The listing builds one solid part. Answer for the finished solid, in the listing's coordinates (mm). Face numbers are marked on the shaded views. A direction names the side the tool comes from. Coordinates: 2 decimals unless noted, no trailing zeros. Write each loop counter-clockwise with the first axis right and the second up, starting at its lowest first coordinate (ties: lowest second). Pieces come first, ordered by that corner, then holes.
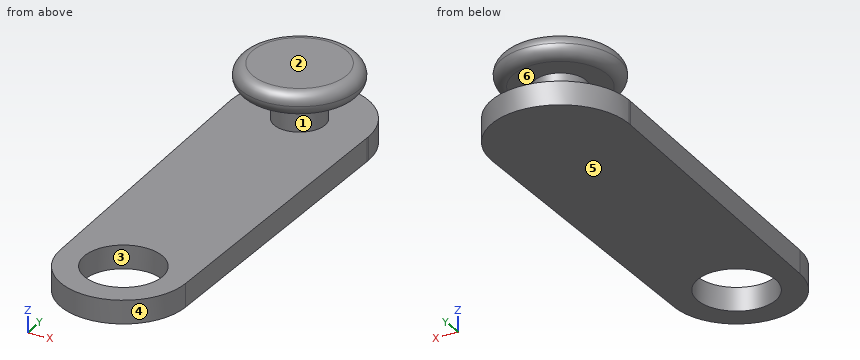
from build123d import *

# Parameters (mm, degrees)
F0_R     = 5
F1_DEPTH = 3
F2_R     = 3.25
F3_DEPTH = 4
F4_R     = 7.5
F5_DEPTH = 3
F6_R     = 1.49999


# Not quite as in the source:
# - a fillet or chamfer is up to 0.001 mm smaller than in the source, because OpenCascade refuses the exact size


with BuildPart() as f1:
    # F0 (on Top) → F1 (new body)
    with BuildSketch(Plane.XY):
        with BuildLine():
            Line((8.8034559258, 0), (8.7968361379, -0.3413359058))
            ThreePointArc((8.7968361379, -0.3413359058), (8.8018008233, -0.1707000455), (8.8034559258, 0))
        make_face()
        with BuildLine():
            Line((8.024687147, -40.1556288865), (8.7968361379, -0.3413359058))
            Line((8.7968361379, -0.3413359058), (8.8034559258, 0))
            ThreePointArc((8.8034559258, 0), (0, 8.8034559258), (-8.8034559258, 0))
            Line((-8.8034559258, 0), (-8.7968361379, -0.3413359058))
            Line((-8.7968361379, -0.3413359058), (-8.024687147, -40.1556288865))
            ThreePointArc((-8.024687147, -40.1556288865), (0, -48.02619612), (8.024687147, -40.1556288865))
        make_face()
        with Locations((0, -40)):
            Circle(F0_R, mode=Mode.SUBTRACT)
        with BuildLine():
            Line((-8.7968361379, -0.3413359058), (-8.8034559258, 0))
            ThreePointArc((-8.8034559258, 0), (-8.8018008233, -0.1707000455), (-8.7968361379, -0.3413359058))
        make_face()
    extrude(amount=F1_DEPTH)

    # F2 (on face) → F3 (join)
    with BuildSketch(Plane.XY.offset(3)):
        Circle(F2_R)
    extrude(amount=F3_DEPTH)

    # F4 (on face) → F5 (join)
    with BuildSketch(Plane.XY.offset(7)):
        Circle(F4_R)
    extrude(amount=F5_DEPTH)

    # F6 (radius 1.5 in the source; OpenCascade refuses exactly that, so slightly less here)
    f6_edges = [f1.edges().sort_by_distance(p)[0] for p in [
        (-7.5, 0, 10),
        (-7.5, 0, 7),
    ]]
    fillet(f6_edges, radius=F6_R)


solid = f1.part
1. For a pull along Y with two mould halves and no side action, classify the marked faces 1, 2, 3 and 4 as pulls with the +Y half, pulls with the -Y half, needs draft (parallel to the pull), parting line crosses it, or undercut.
Results found:
face 1: parting line crosses it
face 2: needs draft
face 3: undercut
face 4: pulls with the -Y half
2. A tool of negligible diameter and unlimited length cuts with its end or side. For the marked faces 5 and 6, from which of +Z, -Z, +X, -X, +Y, -Y can it reach the whole face along a straight path? Write none if from no direction.
Results found:
face 5: -Z, +X, -X, +Y, -Y
face 6: none
3. Section C-C on y = -34.5 is taken. Give the vertices of the cut face in (x, z).
Results found:
outline: (-8.13, 0) - (8.13, 0) - (8.13, 3) - (-8.13, 3) - close
4. Flat-ended cylindrical pins translate along their axes: P1, Ø4, axis at x = 1.5, z = 7, coming from the -Y side; P2, Ø9, axis at x = 0, y = -20.5, coming from the +Z side; P3, Ø1, axis at x = -5, z = 2.5, coming from the +Y side; P4, Ø3, axis at x = 7, y = -18, coming from the -Z side. Find the tip coordinate at first contact, or state that the pin passes through.
Results found:
P1: stops at y = -7.5
P2: stops at z = 3
P3: stops at y = 7.57
P4: stops at z = 0
5. Section D-D on z = 5.25 is taken. Give the vertices of the cut face in (x, y), then the cut area to 3 significant figures.
Results found:
outline: circle Ø6.5 at (0, 0)
area: 33.2 mm2
6. Find the intervals of material crossed by L1, parallel to Z at x = -8, y = -36; L2, parallel to Z at x = 3.5, y = 4; L3, parallel to Y at x = -3, z = 1, in increasing order.
Results found:
L1: z = 0 to 3
L2: z = 0 to 3, 7 to 10
L3: y = -47.44 to -44, -36 to 8.28
